Source: CAD feature listing. Evaluate the final solid. Frame: model axes, mm. A direction names the side the tool comes from. Round coordinates to 2 decimals unless told otherwise and drop trailing zeros. Write each loop counter-clockwise with the first axis right and the second up, starting at its lowest first coordinate (ties: lowest second). Pieces come first, ordered by that corner, then holes. Notation, with made-up numbers: M 85,-36 L 117,-36 A26 ccw 117,-5 Z; hole C -38,19 d7. An arc over 180 degrees is marked long. Use a Markdown table: item, result.
Autodesk Inventor part; units mm, degrees
ref_plane "YZ Plane" through (0, 0, 0) normal (1, 0, 0) x (0, 1, 0)
ref_plane "XZ Plane" through (0, 0, 0) normal (0, 1, 0) x (-1, 0, 0)
ref_plane "XY Plane" through (0, 0, 0) normal (0, 0, 1) x (1, 0, 0)
sketch "Sketch1" plane through (0, 0, 0) normal (0, 1, 0) x (-1, 0, 0)
  line L0 (0, 0) -> (60, 0)
  line L1 (60, 0) -> (60, -40)
  line L2 (60, -40) -> (0, -40)
  line L3 (0, -40) -> (0, 0)
  line L4 (0, -20) -> (60, -20)
  line L5 (0, 0) -> (0, -20)
  line L6 (0, -10) -> (7.5, -10)
  line L7 (0, -10) -> (7.5, -10) construction
  circle A0 centre (7.5, -10) radius 2.5
  line L8 (60, -10) -> (52.5, -10)
  circle A1 centre (52.5, -10) radius 2.5
  circle A2 centre (7.5, -30) radius 2.5
  circle A3 centre (52.5, -30) radius 2.5
  dimension "d0" = 60
  dimension "d1" = 40
  dimension "d2" = 7.5
  dimension "d3" = 0
  dimension "d4" = 5
  dimension "d5" = 7.5
  dimension "d6" = 5
extrude "Extrusion1" add sketch "Sketch1" along normal blind 5.08
ref_plane "Work Plane1" through (-30, 0, -40) normal (-1, 0, 0) x (0, 0, 1)
sketch "Sketch2" plane through (-30, 0, -40) normal (-1, 0, 0) x (0, 0, 1)
  line L0 (40, 0) -> (0, 0)
  line L1 (0, 0) -> (0, 5.08)
  line L2 (40, 5.08) -> (0, 5.08)
  line L3 (40, 0) -> (40, 5.08)
  line L4 (0, 0) -> (40, 0)
  line L5 (20, 0) -> (20, 25.4)
  line L6 (20, 25.4) -> (20, 15.24)
  line L7 (7.3, 5.08) -> (32.7, 5.08)
  line L8 (32.7, 5.08) -> (32.7, 25.4)
  line L9 (32.7, 25.4) -> (7.3, 25.4)
  line L10 (7.3, 25.4) -> (7.3, 5.08)
  line L11 (7.3, 5.08) -> (32.7, 25.4) construction
  line L12 (32.7, 5.08) -> (7.3, 25.4) construction
  dimension "d9" = 25.4
  dimension "d10" = 10.16
  dimension "d11" = 25.4
extrude "Extrusion2" add sketch "Sketch2" along normal mid plane 30.48 contours L5 L9 L8 L2 | L2 L10 L9 L5
sketch "Sketch3" plane through (-45.24, 25.4, -32.7) normal (0, 1, 0) x (1, 0, 0)
  line L0 (30.48, 0) -> (0, 0)
  line L1 (0, -25.4) -> (0, 0)
  line L2 (30.48, -25.4) -> (0, -25.4)
  line L3 (30.48, 0) -> (30.48, -25.4)
  line L4 (17.4625, -1.27) -> (13.0175, -1.27)
  line L5 (13.0175, -1.27) -> (13.0175, -24.13)
  line L6 (13.0175, -24.13) -> (17.4625, -24.13)
  line L7 (17.4625, -24.13) -> (17.4625, -1.27)
  line L8 (17.4625, -1.27) -> (13.0175, -24.13) construction
  line L9 (13.0175, -1.27) -> (17.4625, -24.13) construction
  line L10 (27.94, -6.985) -> (2.54, -6.985)
  line L11 (2.54, -6.985) -> (2.54, -18.415)
  line L12 (2.54, -18.415) -> (27.94, -18.415)
  line L13 (27.94, -18.415) -> (27.94, -6.985)
  line L14 (27.94, -6.985) -> (2.54, -18.415) construction
  line L15 (2.54, -6.985) -> (27.94, -18.415) construction
  point P0 (45.24, -32.7)
  point P1 (15.24, -12.7)
  point P2 (15.24, -12.7)
  dimension "d14" = 4.445
  dimension "d15" = 22.86
  dimension "d16" = 25.4
  dimension "d17" = 11.43
extrude "Extrusion3" cut sketch "Sketch3" against normal blind 20.32 contours L7 L10 L5 L4 | L10 L13 L12 L7 | L7 L12 L5 L10 | L5 L12 L11 L10 | L7 L6 L5 L12
fillet "Fillet1" radius 5.08 4 edges at (-37.4613, 5.08, -25.715) (-37.4613, 5.08, -14.285) (-22.5388, 5.08, -14.285) (-22.5388, 5.08, -25.715)
fillet "Fillet2" radius 10.16 2 edges at (-30, 5.08, -31.43) (-30, 5.08, -8.57)
sketch "Sketch4" plane through (-42.7, 25.4, -14.285) normal (1, 0, 0) x (0, 0, -1)
  arc A0 (0, -15.24) -> (5.08, -20.32) centre (5.08, -15.24) ccw
  line L0 (5.08, -20.32) -> (6.35, -20.32)
  arc A1 (6.35, -20.32) -> (11.43, -15.24) centre (6.35, -15.24) ccw
  line L1 (11.43, 0) -> (11.43, -15.24)
  line L2 (0, 0) -> (11.43, 0)
  line L3 (0, 0) -> (0, -15.24)
  line L4 (5.715, 0) -> (5.715, -10.16)
  line L5 (5.715, 0) -> (15.875, 0) construction
  circle A2 centre (5.715, -10.16) radius 5
  point P0 (-14.285, -25.4)
  dimension "d22" = 10.16
  dimension "d23" = 90
  dimension "d24" = 10
extrude "Extrusion4" cut sketch "Sketch4" along normal mid plane 117.1575 contours A2
sketch "Sketch5" plane through (0, 0, -40) normal (0, 0, -1) x (-1, 0, 0)
  line L0 (10, 0) -> (10, 5.08)
  line L1 (0, 0) -> (60, 0)
  line L2 (60, 0) -> (60, 5.08)
  line L3 (0, 5.08) -> (60, 5.08)
  line L4 (0, 0) -> (0, 5.08)
  line L5 (45.24, 5.08) -> (14.76, 5.08)
  line L6 (45.24, 25.4) -> (45.24, 5.08)
  line L7 (14.76, 25.4) -> (45.24, 25.4)
  line L8 (14.76, 5.08) -> (14.76, 25.4)
  line L9 (14.76, 25.4) -> (0, 5.08)
  line L10 (45.24, 5.08) -> (45.24, 25.4)
  line L11 (45.24, 25.4) -> (60, 5.08)
extrude "Extrusion5" add sketch "Sketch5" along normal blind 5.08
sketch "Sketch6" plane through (-14.76, 5.08, -32.7) normal (0, 0, -1) x (-1, 0, 0)
  line L0 (13.0175, 0) -> (2.54, 0)
  line L1 (30.48, 0) -> (0, 0)
  line L2 (30.48, 20.32) -> (30.48, 0)
  line L3 (0, 20.32) -> (30.48, 20.32)
  line L4 (0, 0) -> (0, 20.32)
  point P0 (-14.76, -5.08)
extrude "Extrusion6" add sketch "Sketch6" along normal up to surface (7.3 mm away)
ref_plane "Work Plane2" through (-27.7775, 25.4, -20) normal (0, 0, 1) x (1, 0, 0)
mirror "Mirror1" about plane through (-27.7775, 25.4, -20) normal (0, 0, 1) of "Extrusion5", "Extrusion6"
properties part number "Ythruster"
Q1. Section D-D on x = -23.5. Return loops of the section in (y, z) (3 decimals).
Results are:
| item | result |
|---|---|
| outline | M 0,-45.08 L 25.4,-45.08 L 25.4,-25.715 L 10.16,-25.715 A5.08 cw 5.08,-20.635 L 5.08,-19.365 A5.08 cw 10.16,-14.285 L 25.4,-14.285 L 25.4,5.08 L 0,5.08 Z |
Q2. Line query: L1, parallel to Z at x = -7.5, y = 3.85; L2, parallel to Y at x = -15.35, z = -20; L3, parallel to Z at x = -35, y = 23.5 (3 decimals). Output: solid intervals per line, ascending.
Results are:
| item | result |
|---|---|
| L1 | -45.08 to -32.5, -27.5 to -12.5, -7.5 to 5.08 |
| L2 | 0 to 10.24, 20.24 to 25.4 |
| L3 | -45.08 to -25.715, -14.285 to 5.08 |
Q3. Section A-A on y = 3.5. Return loops of the section in (x, z).
Results are:
| item | result |
|---|---|
| outline | M -60,-45.08 L 0,-45.08 L 0,5.08 L -60,5.08 Z; hole C -52.5,-30 d5; hole C -52.5,-10 d5; hole C -7.5,-30 d5; hole C -7.5,-10 d5 |
Q4. Section C-C on x = -6. Return loops of the section in (y, z).
Results are:
| item | result |
|---|---|
| outline | M 0,-45.08 L 13.34,-45.08 L 13.34,-40 L 5.08,-40 L 5.08,-32 L 0,-32 Z; M 0,-28 L 5.08,-28 L 5.08,-12 L 0,-12 Z; M 0,-8 L 5.08,-8 L 5.08,0 L 13.34,0 L 13.34,5.08 L 0,5.08 Z |
Q5. Section B-B on z = -24. Return loops of the section in (x, y).
Results are:
| item | result |
|---|---|
| outline | M -60,0 L 0,0 L 0,5.08 L -14.76,5.08 L -14.76,12.24 L -17.3,12.24 L -17.3,6.35 L -27.78,6.35 L -27.78,5.45 L -32.22,5.45 L -32.22,6.35 L -42.7,6.35 L -42.7,12.24 L -45.24,12.24 L -45.24,5.08 L -60,5.08 Z; M -45.24,18.24 L -42.7,18.24 L -42.7,25.4 L -45.24,25.4 Z; M -17.3,18.24 L -14.76,18.24 L -14.76,25.4 L -17.3,25.4 Z |
Q6. First-contact query: pin 1 Ø6 at (y, z) = (8, -25.5) entering from -X; pin 2 Ø5.5 at (y, z) = (18.5, -23.5) entering from +X; pin 3 Ø9 at (y, z) = (16, -22) entering from -X; pin 4 Ø7.5 at (x, z) = (-10, -10.5) entering from +Y. Flat tips, straight axial feed; report the tip coordinate or a pass-through.
Results are:
| item | result |
|---|---|
| pin 1 | x = -60 |
| pin 2 | x = -14.76 |
| pin 3 | x = -45.24 |
| pin 4 | y = 5.08 |
Q7. Mould query, pull axis Y, two halves, no side actions, for faces 1 (the cylindrical face through (-22.47, 6.61, -15.73)), 2 (the flat face through (-30, 10, -45.08)), 3 (the cylindrical face through (-43.99, 20.12, -18.92)), 4 (the flat face through (-30, 0, -20)). Classes: +Y half, -Y half, draft (parallel to the pull), parting line (faces both ways), or undercut.
Results are:
| item | result |
|---|---|
| face 1 | +Y half |
| face 2 | draft |
| face 3 | undercut |
| face 4 | -Y half |
Q8. Reachability of faces 5 (the flat face through (-37, 18, -25.715)), 6 (the flat face through (-14.76, 18, -25)), 7 (the flat face through (-49, 11, -40)) from +Z, -Z, +X, -X, +Y, -Y: full face, straight path, thin tool, end or side. Return the list, or none.
Results are:
| item | result |
|---|---|
| face 5 | +Y |
| face 6 | +X, +Y |
| face 7 | -X, +Y |
